```python
from build123d import *

# Parameters (mm, degrees)
BOSS_EXTRUDE1_DEPTH = 25.4
SKETCH5_R           = 3.429
CUT_EXTRUDE1_DEPTH  = 1.5875
SKETCH6_R           = 1.27
CUT_EXTRUDE2_DEPTH  = 29.93651842


with BuildPart() as part:
    # Sketch4 → Boss-Extrude1 (new, symmetric)
    with BuildSketch(Plane(origin=(0, 0, 0), x_dir=(1, 0, 0), z_dir=(0, 1, 0))):
        with BuildLine():
            Line((94.399536545, 12.7), (88.106234109, 11.853333333))
            ThreePointArc((88.106234109, 11.853333333), (88.9, 0), (88.106234109, -11.853333333))
            Line((88.106234109, -11.853333333), (94.399536545, -12.7))
            ThreePointArc((94.399536545, -12.7), (95.25, 0), (94.399536545, 12.7))
        make_face()
    extrude(amount=BOSS_EXTRUDE1_DEPTH, both=True)

    # Sketch5 → Cut-Extrude1 (cut)
    with BuildSketch(Plane(origin=(95.25, 25.4, 0), x_dir=(0, 0, -1), z_dir=(1, 0, 0))):
        with Locations((0, -25.4)):
            Circle(SKETCH5_R)
    extrude(amount=-CUT_EXTRUDE1_DEPTH, mode=Mode.SUBTRACT)

    # Sketch6 → Cut-Extrude2 (cut, through all)
    with BuildSketch(Plane(origin=(93.6625, 0, 0), x_dir=(0, 0, -1), z_dir=(1, 0, 0))):
        Circle(SKETCH6_R)
    extrude(amount=-CUT_EXTRUDE2_DEPTH, mode=Mode.SUBTRACT)


solid = part.part
```
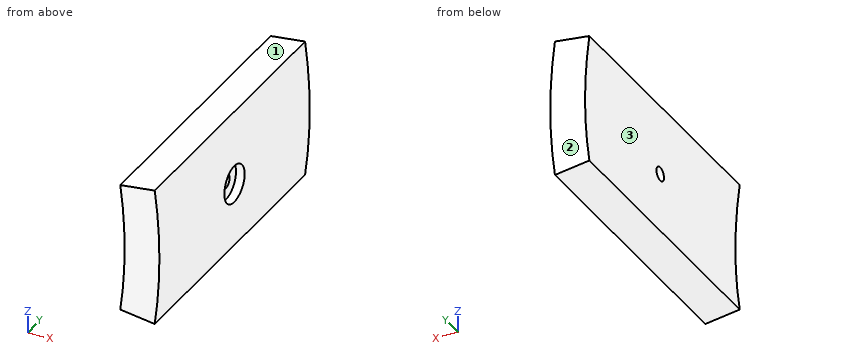
The listing builds one solid part. Answer for the finished solid, in the listing's coordinates (mm). Face numbers are marked on the shaded views. Coordinates: 2 decimals unless noted, no trailing zeros. Write each loop counter-clockwise with the first axis right and the second up, starting at its lowest first coordinate (ties: lowest second). Pieces come first, ordered by that corner, then holes. Notation, with made-up numbers: (-6, 62.5) -> (25, 62.5) arc R34 cw to (25, 100.5) -> close; hole circle Ø6 at (64, 24.25). An arc over 180 degrees is marked (long way). Write each question's results on one line, items separated by ' | '. Start each with the question number.
1) Flat-ended cylindrical pins translate along their axes: pin 1 Ø3.5 at (y, z) = (0, 0) entering from -X; pin 2 Ø1 at (x, y) = (92, 7) entering from +Z; pin 3 Ø8 at (y, z) = (17.5, -5) entering from +X. Find the tip coordinate at first contact, or state that the pin passes through.
2) A cutting plane is placed at D-D (y = 9). Determine the outline of the cut face in (x, z).
3) For a pull along Z with two mould halves and no side action, classify the marked faces 1, 2 and 3 as +Z half, -Z half, draft (parallel to the pull), parting line (faces both ways), or undercut.
4) A cutting plane is placed at B-B (z = 0). Determine the outline of the cut face in (x, y), then the cut area to 3 significant figures.
5) Straight lines are drawn through the part: probe 1 along Y at (x, z) = (94.2, 0); probe 2 along Y at (x, z) = (91.8, 0); probe 3 along X at (y, z) = (-2, -0.5). For each, find the intervals that lie inside material, in ascending order.
6) A cutting plane is placed at A-A (y = 0). Determine the outline of the cut face in (x, z).
7) A cutting plane is placed at C-C (x = 90). Determine the outline of the cut face in (y, z).
Values follow:
1) pin 1: x = 88.88 | pin 2: z = 12.44 | pin 3: x = 95.24
2) outline: (88.11, -11.85) -> (94.4, -12.7) arc R95.25 ccw to (94.4, 12.7) -> (88.11, 11.85) arc R88.9 cw to start
3) face 1: +Z half | face 2: draft | face 3: undercut
4) outline: (88.9, -25.4) -> (95.25, -25.4) -> (95.25, -3.43) -> (93.66, -3.43) -> (93.66, -1.27) -> (88.9, -1.27) -> close; (88.9, 1.27) -> (93.66, 1.27) -> (93.66, 3.43) -> (95.25, 3.43) -> (95.25, 25.4) -> (88.9, 25.4) -> close | area: 300 mm²
5) probe 1: -25.4 to -3.43, 3.43 to 25.4 | probe 2: -25.4 to -1.27, 1.27 to 25.4 | probe 3: 88.9 to 93.66
6) outline: (88.11, -11.85) -> (94.4, -12.7) arc R95.25 ccw to (95.19, -3.43) -> (93.66, -3.43) -> (93.66, -1.27) -> (88.89, -1.27) arc R88.9 cw to start; (88.11, 11.85) arc R88.9 cw to (88.89, 1.27) -> (93.66, 1.27) -> (93.66, 3.43) -> (95.19, 3.43) arc R95.25 ccw to (94.4, 12.7) -> close
7) outline: (-25.4, -12.11) -> (25.4, -12.11) -> (25.4, 12.11) -> (-25.4, 12.11) -> close; hole circle Ø2.54 at (0, 0)
